Work out the finished part from the listing and answer in its coordinate system (mm). A direction names the side the tool comes from. Give positions to 0.01 mm unless a question says otherwise; leave off trailing zeros. Loops run counter-clockwise (first coordinate to the right, second up) from the corner with the lowest first, then second, coordinate; pieces in that order, holes last. Notation, with made-up numbers: M -3,-20.75 L 40,-20.75 A27 ccw 40,1.25 Z; hole C 58.5,76.5 d11. An arc over 180 degrees is marked long. Write item = value, one per line. Start each with the question number.
1. For faces 4 (the face through (-3.49, 18.78, 3.63)), 5 (the face through (38, 25.4, -98)), determine the directions among +Z, -Z, +X, -X, +Y, -Y from which every point of the face is accessible in a straight line to the end or side of a thin tool.
2. Section A-A on z = -22 is taken. Determine the outline of the cut face in (x, y) (3 decimals), plus the area to 3 significant figures.
3. Flat-ended cylindrical pins translate along their axes: pin 1 Ø1.6 at (x, z) = (40.5, -9.5) entering from +Y (3 decimals); pin 2 Ø4 at (y, z) = (9.5, 4) entering from +X; pin 3 Ø8.5 at (x, z) = (39.5, -8.5) entering from +Y (3 decimals). Find the tip coordinate at first contact, or state that the pin passes through.
4. Section B-B on y = 17 is taken. Determine the outline of the cut face in (x, z) (3 decimals).
5. Section C-C on x = 67 is taken. Determine the outline of the cut face in (y, z) (3 decimals).
6. The mould has two halves that part along Y. Classify faces 1 (the face through (38, 21, -93.175)), 2 (the face through (29.688, 9, 2)), 3 (the face through (-2, 25.4, -48)): released by +Y, released by -Y, zero draft, split by the parting line, or undercut.
7. Consider L1, parallel to Z at x = 52, y = 16.5 (3 decimals); L2, parallel to X at y = 31.5, z = -92 (3 decimals); L3, parallel to X at y = 32, z = -47 (3 decimals). Determine where each line is inside the solid, lowest interval first. Write a range as [from, to].
```python
from build123d import *

# Parameters (mm, degrees)
BOSS_EXTRUDE1_DEPTH = 38.1
SKETCH2_W           = 69.999999954
SKETCH2_H           = 90.000000086
CUT_EXTRUDE1_DEPTH  = 34.925
SKETCH3_R           = 3.96875
SKETCH3_R_2         = 1.5875
BOSS_EXTRUDE2_DEPTH = 10.16
BOSS_EXTRUDE3_DEPTH = 38.1
SKETCH5_R           = 1.5875
CUT_EXTRUDE2_DEPTH  = 12.7
SKETCH7_W           = 12
SKETCH7_H           = 8
CUT_EXTRUDE3_DEPTH  = 9.525


with BuildPart() as part:
    # Sketch1 → Boss-Extrude1 (new body)
    with BuildSketch(Plane(origin=(0, 0, 0), x_dir=(1, 0, 0), z_dir=(0, 1, 0))):
        with BuildLine():
            Line((3.175, 0), (73.174999954, 0))
            ThreePointArc((73.174999954, 0), (75.420063984, 0.92993597), (76.349999954, 3.175))
            Line((76.349999954, 3.175), (76.349999954, 93.175000086))
            ThreePointArc((76.349999954, 93.175000086), (75.420063984, 95.420064116), (73.174999954, 96.350000086))
            Line((73.174999954, 96.350000086), (3.175, 96.350000086))
            ThreePointArc((3.175, 96.350000086), (0.92993597, 95.420064116), (0, 93.175000086))
            Line((0, 93.175000086), (0, 3.175))
            ThreePointArc((0, 3.175), (0.92993597, 0.92993597), (3.175, 0))
        make_face()
    extrude(amount=BOSS_EXTRUDE1_DEPTH)

    # Sketch2 → Cut-Extrude1 (cut)
    with BuildSketch(Plane(origin=(0, 38.1, 0), x_dir=(1, 0, 0), z_dir=(0, 1, 0))):
        with Locations((38.174999977, 48.175000043)):
            Rectangle(SKETCH2_W, SKETCH2_H)
    extrude(amount=-CUT_EXTRUDE1_DEPTH, mode=Mode.SUBTRACT)

    # Sketch3 → Boss-Extrude2 (add)
    # profile 1 of 2: a face of its own
    with BuildSketch(Plane(origin=(0, 3.175, 0), x_dir=(1, 0, 0), z_dir=(0, 1, 0))):
        with Locations(Location((21.587999977, 88.875000043, 0), (0, 0, 90))):
            Circle(SKETCH3_R)
        with Locations(Location((21.587999977, 88.875000043, 0), (0, 0, 270))):
            Circle(SKETCH3_R_2, mode=Mode.SUBTRACT)
    # profile 2 of 2: a face of its own
    with BuildSketch(Plane(origin=(0, 3.175, 0), x_dir=(1, 0, 0), z_dir=(0, 1, 0))):
        with Locations(Location((39.987999977, 9.175000043, 0), (0, 0, 90))):
            Circle(SKETCH3_R)
        with Locations(Location((39.987999977, 9.175000043, 0), (0, 0, 270))):
            Circle(SKETCH3_R_2, mode=Mode.SUBTRACT)
    extrude(amount=BOSS_EXTRUDE2_DEPTH)

    # Sketch4 → Boss-Extrude3 (add)
    with BuildSketch(Plane.XZ):
        with BuildLine():
            Line((-6.35, -3.175), (-6.35, -93.175000086))
            ThreePointArc((-6.35, -93.175000086), (-3.560192091, -99.910192177), (3.175, -102.700000086))
            Line((3.175, -102.700000086), (73.174999954, -102.700000086))
            ThreePointArc((73.174999954, -102.700000086), (79.910192045, -99.910192177), (82.699999954, -93.175000086))
            Line((82.699999954, -93.175000086), (82.699999954, -3.175))
            ThreePointArc((82.699999954, -3.175), (79.910192045, 3.560192091), (73.174999954, 6.35))
            Line((73.174999954, 6.35), (3.175, 6.35))
            ThreePointArc((3.175, 6.35), (-3.560192091, 3.560192091), (-6.35, -3.175))
        make_face()
        with BuildLine():
            Line((0, -3.175), (0, -93.175000086))
            ThreePointArc((0, -93.175000086), (0.92993597, -95.420064116), (3.175, -96.350000086))
            Line((3.175, -96.350000086), (73.174999954, -96.350000086))
            ThreePointArc((73.174999954, -96.350000086), (75.420063984, -95.420064116), (76.349999954, -93.175000086))
            Line((76.349999954, -93.175000086), (76.349999954, -3.175))
            ThreePointArc((76.349999954, -3.175), (75.420063984, -0.92993597), (73.174999954, 0))
            Line((73.174999954, 0), (3.175, 0))
            ThreePointArc((3.175, 0), (0.92993597, -0.92993597), (0, -3.175))
        make_face(mode=Mode.SUBTRACT)
    extrude(amount=-BOSS_EXTRUDE3_DEPTH)

    # Sketch5 → Cut-Extrude2 (cut)
    with BuildSketch(Plane(origin=(0, 38.1, 0), x_dir=(1, 0, 0), z_dir=(0, 1, 0))):
        with Locations(Location((-1.5875, 48.175000043, 0), (0, 0, 270))):
            Circle(SKETCH5_R)
        with Locations(Location((38.174999977, 97.937500086, 0), (0, 0, 270))):
            Circle(SKETCH5_R)
        with Locations(Location((38.174999977, -1.5875, 0), (0, 0, 90))):
            Circle(SKETCH5_R)
        with Locations(Location((77.937499954, 48.175000043, 0), (0, 0, 90))):
            Circle(SKETCH5_R)
    extrude(amount=-CUT_EXTRUDE2_DEPTH, mode=Mode.SUBTRACT)

    # Sketch7 → Cut-Extrude3 (cut)
    with BuildSketch(Plane.XY.offset(6.35)):
        with Locations((23.687999977, 8.835)):
            Rectangle(SKETCH7_W, SKETCH7_H)
    extrude(amount=-CUT_EXTRUDE3_DEPTH, mode=Mode.SUBTRACT)


solid = part.part
```
Verdict:
q1.face_4 = +Z, -X, +Y, -Y
q1.face_5 = +Y
q2.outline = M -6.35,0 L 82.7,0 L 82.7,38.1 L 73.175,38.1 L 73.175,3.175 L 3.175,3.175 L 3.175,38.1 L -6.35,38.1 Z
q2.area = 948 mm2
q3.pin_1 = 3.175
q3.pin_2 = 81.17
q3.pin_3 = 13.335
q4.outline = M -6.35,-93.175 A9.525 ccw 3.175,-102.7 L 73.175,-102.7 A9.525 ccw 82.7,-93.175 L 82.7,-3.175 A9.525 ccw 73.175,6.35 L 3.175,6.35 A9.525 ccw -6.35,-3.175 Z; hole M 3.175,-93.175 L 73.175,-93.175 L 73.175,-3.175 L 3.175,-3.175 Z
q5.outline = M 0,-102.7 L 38.1,-102.7 L 38.1,-93.175 L 3.175,-93.175 L 3.175,-3.175 L 38.1,-3.175 L 38.1,6.35 L 0,6.35 Z
q6.face_1 = zero draft
q6.face_2 = undercut
q6.face_3 = released by +Y
q7.L1 = [-102.7, -93.175], [-3.175, 6.35]
q7.L2 = [-6.35, 3.175], [73.175, 82.7]
q7.L3 = [-6.35, -2.655], [-0.52, 3.175], [73.175, 76.87], [79.005, 82.7]
